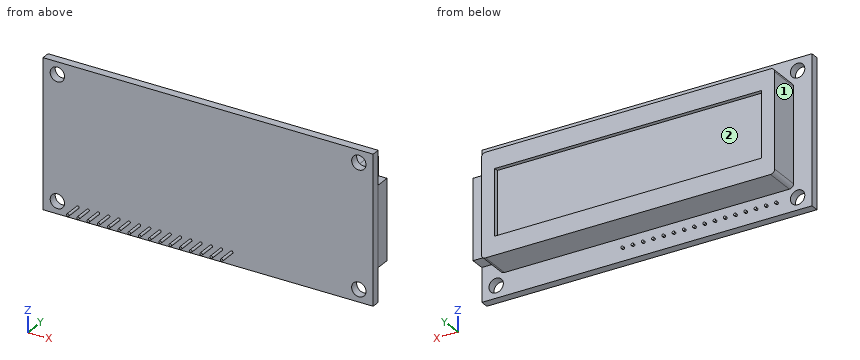
from build123d import *

# Parameters (mm, degrees)
SKETCH1_W                = 80.5
SKETCH1_H                = 36
BOSS_EXTRUDE1_DEPTH      = 2
SKETCH2_R                = 1.75
CUT_EXTRUDE1_DEPTH       = 2
SKETCH3_W                = 71.5
SKETCH3_H                = 25
BOSS_EXTRUDE2_DEPTH      = 7.5
SKETCH4_W                = 65
SKETCH4_H                = 16
CUT_EXTRUDE2_DEPTH       = 1
FILLET1_R                = 1
SKETCH5_W                = 4.5
SKETCH5_H                = 19.5
BOSS_EXTRUDE3_DEPTH      = 3.5
SKETCH6_W                = 19.5
SKETCH6_H                = 3.5
BOSS_EXTRUDE4_DEPTH      = 0.001
BOSS_EXTRUDE5_DEPTH      = 4
BOSS_EXTRUDE5_DEPTH_BACK = 2.5
SKETCH7_R                = 0.3125


with BuildPart() as part:
    # Sketch1 → Boss-Extrude1 (new body)
    with BuildSketch(Plane(origin=(0, 0, 0), x_dir=(1, 0, 0), z_dir=(0, 1, 0))):
        with Locations((-3.238505747, 7.445402299)):
            Rectangle(SKETCH1_W, SKETCH1_H)
    extrude(amount=BOSS_EXTRUDE1_DEPTH)

    # Sketch2 → Cut-Extrude1 (cut)
    with BuildSketch(Plane(origin=(0, 2, 0), x_dir=(1, 0, 0), z_dir=(0, 1, 0))):
        with Locations(Location((-39.988505747, 22.445402299, 0), (0, 0, 270))):
            Circle(SKETCH2_R)
        with Locations(Location((33.511494253, 22.445402299, 0), (0, 0, 270))):
            Circle(SKETCH2_R)
        with Locations(Location((33.511494253, -7.554597701, 0), (0, 0, 270))):
            Circle(SKETCH2_R)
        with Locations(Location((-39.988505747, -7.554597701, 0), (0, 0, 270))):
            Circle(SKETCH2_R)
    extrude(amount=-CUT_EXTRUDE1_DEPTH, mode=Mode.SUBTRACT)

    # Sketch3 → Boss-Extrude2 (add)
    with BuildSketch(Plane(origin=(0, 2, 0), x_dir=(1, 0, 0), z_dir=(0, 1, 0))):
        with Locations((-3.238505747, 7.445402299)):
            Rectangle(SKETCH3_W, SKETCH3_H)
    extrude(amount=BOSS_EXTRUDE2_DEPTH)

    # Sketch4 → Cut-Extrude2 (cut)
    with BuildSketch(Plane(origin=(0, 9.5, 0), x_dir=(1, 0, 0), z_dir=(0, 1, 0))):
        with Locations((-3.238505747, 7.445402299)):
            Rectangle(SKETCH4_W, SKETCH4_H)
    extrude(amount=-CUT_EXTRUDE2_DEPTH, mode=Mode.SUBTRACT)

    # Fillet1
    fillet1_edges = [part.edges().sort_by_distance(p)[0] for p in [
        (-38.988505747, 5.75, -19.945402299),
        (-38.988505747, 5.75, 5.054597701),
        (32.511494253, 5.75, 5.054597701),
        (32.511494253, 5.75, -19.945402299),
    ]]
    fillet(fillet1_edges, radius=FILLET1_R)

    # Sketch5 → Boss-Extrude3 (add)
    with BuildSketch(Plane(origin=(0, 2, 0), x_dir=(1, 0, 0), z_dir=(0, 1, 0))):
        with Locations((34.761494253, 7.445402299)):
            Rectangle(SKETCH5_W, SKETCH5_H)
    extrude(amount=BOSS_EXTRUDE3_DEPTH)

    # Sketch6 → Boss-Extrude4 (add)
    with BuildSketch(Plane(origin=(37.011494253, 0, 0), x_dir=(0, 0, -1), z_dir=(1, 0, 0))):
        with Locations((7.445402299, 3.75)):
            Rectangle(SKETCH6_W, SKETCH6_H)
    extrude(amount=BOSS_EXTRUDE4_DEPTH)

    # Sketch7 → Boss-Extrude5 (add, two sides: drawn at the far end of the back side and taken through both)
    with BuildSketch(Plane(origin=(0, 0, 0), x_dir=(-1, 0, 0), z_dir=(0, -1, 0)).offset(-BOSS_EXTRUDE5_DEPTH_BACK)):
        with Locations(Location((34.988505747, 22.445402299, 0), (0, 0, 90))):
            Circle(SKETCH7_R)
        with Locations(Location((32.488505747, 22.445402299, 0), (0, 0, 90))):
            Circle(SKETCH7_R)
        with Locations(Location((29.988505747, 22.445402299, 0), (0, 0, 90))):
            Circle(SKETCH7_R)
        with Locations(Location((27.488505747, 22.445402299, 0), (0, 0, 90))):
            Circle(SKETCH7_R)
        with Locations(Location((24.988505747, 22.445402299, 0), (0, 0, 90))):
            Circle(SKETCH7_R)
        with Locations(Location((22.488505747, 22.445402299, 0), (0, 0, 90))):
            Circle(SKETCH7_R)
        with Locations(Location((19.988505747, 22.445402299, 0), (0, 0, 90))):
            Circle(SKETCH7_R)
        with Locations(Location((17.488505747, 22.445402299, 0), (0, 0, 90))):
            Circle(SKETCH7_R)
        with Locations(Location((14.988505747, 22.445402299, 0), (0, 0, 90))):
            Circle(SKETCH7_R)
        with Locations(Location((12.488505747, 22.445402299, 0), (0, 0, 90))):
            Circle(SKETCH7_R)
        with Locations(Location((9.988505747, 22.445402299, 0), (0, 0, 90))):
            Circle(SKETCH7_R)
        with Locations(Location((7.488505747, 22.445402299, 0), (0, 0, 90))):
            Circle(SKETCH7_R)
        with Locations(Location((4.988505747, 22.445402299, 0), (0, 0, 90))):
            Circle(SKETCH7_R)
        with Locations(Location((2.488505747, 22.445402299, 0), (0, 0, 90))):
            Circle(SKETCH7_R)
        with Locations(Location((-0.011494253, 22.445402299, 0), (0, 0, 90))):
            Circle(SKETCH7_R)
        with Locations(Location((-2.511494253, 22.445402299, 0), (0, 0, 90))):
            Circle(SKETCH7_R)
    extrude(amount=BOSS_EXTRUDE5_DEPTH + BOSS_EXTRUDE5_DEPTH_BACK)


solid = part.part
Here's how the part is built. I have some questions about the finished solid (model axes, mm). Face numbers are marked on the shaded views. Round coordinates to 2 decimals unless told otherwise and drop trailing zeros. Loops run counter-clockwise (first coordinate to the right, second up) from the corner with the lowest first, then second, coordinate; pieces in that order, holes last.
1. If we section it at B-B on z = -18: Write out the boundary of the cut face in (x, y).
Answer list:
outline: (-43.49, 0) - (37.01, 0) - (37.01, 2) - (32.51, 2) - (32.51, 9.5) - (-38.99, 9.5) - (-38.99, 2) - (-43.49, 2) - close
2. If I drill on line 1 along Z through (x, y) = (-12.5, 2.25); line 2 along X through (y, z) = (1, 7); line 3 along X through (y, z) = (9.25, -8.5), over which ranges is the centre line in solid material (lowest first)?
Answer list:
line 1: z = -22.76 to -22.13, -19.95 to 5.05
line 2: x = -43.49 to -41.65, -38.33 to 31.85, 35.17 to 37.01
line 3: x = -38.99 to -35.74, 29.26 to 32.51
3. We'd pull the mould along Z, two halves only. Please class the marked faces 1 and 2: +Z half, -Z half, draft (parallel to the pull), parting line (faces both ways), or undercut.
Answer list:
face 1: draft
face 2: undercut
4. If we section it at C-C on x = 21: Write out the boundary of the cut face in (y, z), plus the area to 4 significant figures.
Answer list:
outline: (0, -25.45) - (2, -25.45) - (2, -19.95) - (9.5, -19.95) - (9.5, -15.45) - (8.5, -15.45) - (8.5, 0.55) - (9.5, 0.55) - (9.5, 5.05) - (2, 5.05) - (2, 10.55) - (0, 10.55) - close
area: 243.5 mm2
5. For P1, Ø4, axis at x = -18.5, y = 4.5, coming from the -Z side; P2, Ø4.5, axis at x = 33.51, z = -22.45, coming from the +Y side; P3, Ø4, axis at x = -39.99, z = 7.55, coming from the -Y side; P4, Ø3, axis at x = 22.5, y = -0.5, coming from the -Z side, each with a flat end and sliding along its axis, tell me the tip position at first contact or that it passes through.
Answer list:
P1: stops at z = -19.95
P2: stops at y = 2
P3: stops at y = 0
P4: stops at z = -25.45
6. If we section it at D-D on y = -3: Count the separate pieces of the cut face and the enclosed holes in it, plus the area to 3 significant figures.
Answer list:
separate pieces: 16
enclosed holes: 0
area: 4.91 mm2
7. If we section it at A-A on y = 6.75: Write out the boundary of the cut face in (x, z).
Answer list:
outline: (-38.99, -18.95) arc R1 ccw to (-37.99, -19.95) - (31.51, -19.95) arc R1 ccw to (32.51, -18.95) - (32.51, 4.05) arc R1 ccw to (31.51, 5.05) - (-37.99, 5.05) arc R1 ccw to (-38.99, 4.05) - close
